```python
from build123d import *

# Parameters (mm, degrees)
SKETCH2_R               = 2.15
BOSS_EXTRUDE1_DEPTH     = 12.7
CUT_EXTRUDE1_DEPTH      = 86.777857097
CUT_EXTRUDE1_DEPTH_BACK = 86.777857097
SKETCH3_W               = 5.08
SKETCH3_H               = 2.54
BOSS_EXTRUDE2_DEPTH     = 12.7
SKETCH5_R               = 9.75
CUT_EXTRUDE2_DEPTH      = 5.5
CUT_EXTRUDE3_DEPTH      = 90.593664183
CUT_EXTRUDE3_DEPTH_BACK = 90.593664183
SKETCH6_R               = 1.25


with BuildPart() as part:
    # Sketch2 → Boss-Extrude1 (new body)
    with BuildSketch(Plane(origin=(0, 0, 0), x_dir=(1, 0, 0), z_dir=(0, 1, 0))):
        with BuildLine():
            Line((0, 8.382), (74.7776, 8.382))
            ThreePointArc((74.7776, 8.382), (83.1596, 0), (74.7776, -8.382))
            Line((74.7776, -8.382), (0, -8.382))
            ThreePointArc((0, -8.382), (-8.382, 0), (0, 8.382))
        make_face()
        with Locations(Location((0, 0, 0), (0, 0, 270))):
            Circle(SKETCH2_R, mode=Mode.SUBTRACT)
        with Locations(Location((74.7776, 0, 0), (0, 0, 270))):
            Circle(SKETCH2_R, mode=Mode.SUBTRACT)
    extrude(amount=-BOSS_EXTRUDE1_DEPTH)

    # Sketch3 → Cut-Extrude1 (cut, two sides: drawn at the far end of the back side and taken through both)
    with BuildSketch(Plane(origin=(0, 0, -8.382), x_dir=(-1, 0, 0), z_dir=(0, 0, -1)).offset(-CUT_EXTRUDE1_DEPTH_BACK)):
        with Locations((-43.750123937, -4.528631303)):
            Rectangle(SKETCH3_W, SKETCH3_H)
    extrude(amount=CUT_EXTRUDE1_DEPTH + CUT_EXTRUDE1_DEPTH_BACK, mode=Mode.SUBTRACT)

    # Sketch4 → Boss-Extrude2 (add)
    with BuildSketch(Plane(origin=(0, 0, 0), x_dir=(1, 0, 0), z_dir=(0, 1, 0))):
        with BuildLine():
            Line((71.377269841, 13.064752382), (70.480233935, 12.79775937))
            ThreePointArc((70.480233935, 12.79775937), (67.016909963, 11.04634284), (64.194969136, 8.382))
            Line((64.194969136, 8.382), (74.7776, 8.382))
            ThreePointArc((74.7776, 8.382), (83.1596, 0), (74.7776, -8.382))
            Line((74.7776, -8.382), (64.194969136, -8.382))
            ThreePointArc((64.194969136, -8.382), (66.930768284, -10.985318931), (70.280616628, -12.728988198))
            ThreePointArc((70.280616628, -12.728988198), (82.573134763, -11.021780154), (88.2776, 0))
            ThreePointArc((88.2776, 0), (83.034280412, 10.680694199), (71.377269841, 13.064752382))
        make_face()
        with BuildLine():
            Line((70.480233935, 12.79775937), (55.644284932, 8.382))
            Line((55.644284932, 8.382), (64.194969136, 8.382))
            ThreePointArc((64.194969136, 8.382), (67.016909963, 11.04634284), (70.480233935, 12.79775937))
        make_face()
        with BuildLine():
            ThreePointArc((70.280616628, -12.728988198), (66.930768284, -10.985318931), (64.194969136, -8.382))
            Line((64.194969136, -8.382), (55.644284932, -8.382))
            Line((55.644284932, -8.382), (70.280616628, -12.728988198))
        make_face()
    extrude(amount=-BOSS_EXTRUDE2_DEPTH)

    # Sketch5 → Cut-Extrude2 (cut)
    with BuildSketch(Plane(origin=(0, -12.7, 0), x_dir=(-1, 0, 0), z_dir=(0, -1, 0))):
        with Locations(Location((-74.7776, 0, 0), (0, 0, 90))):
            Circle(SKETCH5_R)
    extrude(amount=-CUT_EXTRUDE2_DEPTH, mode=Mode.SUBTRACT)

    # Sketch6 → Cut-Extrude3 (cut, two sides: drawn at the far end of the back side and taken through both)
    with BuildSketch(Plane(origin=(0, -7.2, 0), x_dir=(-1, 0, 0), z_dir=(0, -1, 0)).offset(-CUT_EXTRUDE3_DEPTH_BACK)):
        with Locations(Location((-74.876863781, 6.35, 0), (0, 0, 90))):
            Circle(SKETCH6_R)
        with Locations(Location((-68.4276, 0.099263781, 0), (0, 0, 90))):
            Circle(SKETCH6_R)
        with Locations(Location((-74.678336219, -6.35, 0), (0, 0, 90))):
            Circle(SKETCH6_R)
        with Locations(Location((-81.1276, -0.099263781, 0), (0, 0, 90))):
            Circle(SKETCH6_R)
    extrude(amount=CUT_EXTRUDE3_DEPTH + CUT_EXTRUDE3_DEPTH_BACK, mode=Mode.SUBTRACT)


solid = part.part
```
Geometry: final body of the model. Coordinates: model frame, mm. A direction names the side the tool comes from. Give positions to 0.01 mm unless a question says otherwise; leave off trailing zeros. Write each loop counter-clockwise with the first axis right and the second up, starting at its lowest first coordinate (ties: lowest second). Pieces come first, ordered by that corner, then holes.
1. Reachability of faces 4 (the flat face through (27, -6, -8.382)), 5 (the flat face through (46.29, -5, 0)), 6 (the flat face through (39, -12.7, 0)), 7 (the flat face through (74.9, -7.2, 2.3)), 8 (the flat face through (28, -6, 8.382)) from +Z, -Z, +X, -X, +Y, -Y: full face, straight path, thin tool, end or side. Return the list, or none.
2. Pin query (flat end, axial travel): P1, Ø4, axis at x = 42, y = -8.5, coming from the -Z side; P2, Ø2, axis at x = 68.43, z = -0.1, coming from the -Y side; P3, Ø4, axis at x = 40, y = -3.5, coming from the +Z side; P4, Ø2, axis at y = -8, z = -6.5, coming from the +X side. Return the tip coordinate at first contact, or that it passes through.
3. Line query: probe 1 along X at (y, z) = (-9.5, 0); probe 2 along Z at (x, y) = (33.5, -11.75); probe 3 along X at (y, z) = (-3.75, 6.35). Output: solid intervals per line, ascending.
4. Draft query along X for faces 1 (the flat face through (39, 0, 0)), 2 (the cylindrical face through (83, -9.99, -5.24)), 3 (the cylindrical face through (-8.38, -6.26, 0.18)). Return one class per face: released by +X, released by -X, zero draft, split by the parting line, or undercut.
5. Section query B-B, the plane y = -4.25. Return loops of the section in (x, z).
6. Section query A-A, the plane z = 6.35. Return loops of the section in (x, y).
7. Section query C-C, the plane y = -8.75. Return loops of the section in (x, z).
8. Section query D-D, the plane x = 51.5. Return loops of the section in (y, z).
Computed:
1. face 4: -Z, -X, +Y, -Y
1. face 5: +Z, -Z
1. face 6: +Z, -Z, +X, -X, -Y
1. face 7: -Y
1. face 8: +Z, -X, +Y, -Y
2. P1: stops at z = -8.38
2. P2: passes through
2. P3: stops at z = 8.38
2. P4: stops at x = 87.11
3. probe 1: x = -8.38 to -2.15, 2.15 to 65.03, 84.53 to 88.28
3. probe 2: z = -8.38 to 8.38
3. probe 3: x = -5.47 to 41.21, 46.29 to 73.43, 75.93 to 86.69
4. face 1: zero draft
4. face 2: undercut
4. face 3: released by -X
5. outline: (0, -8.38) - (41.21, -8.38) - (41.21, 8.38) - (0, 8.38) arc R8.38 ccw to start; (46.29, -8.38) - (55.64, -8.38) - (71.38, -13.06) arc R13.5 ccw (long way) to (70.28, 12.73) - (55.64, 8.38) - (46.29, 8.38) - close; hole circle Ø4.3 at (0, 0); hole circle Ø2.5 at (68.43, -0.1); hole circle Ø4.3 at (74.78, 0); hole circle Ø2.5 at (74.68, 6.35); hole circle Ø2.5 at (74.88, -6.35); hole circle Ø2.5 at (81.13, 0.1)
6. outline: (-5.47, -12.7) - (67.38, -12.7) - (67.38, -7.2) - (73.43, -7.2) - (73.43, 0) - (-5.47, 0) - close; (75.93, -7.2) - (82.18, -7.2) - (82.18, -12.7) - (86.69, -12.7) - (86.69, 0) - (75.93, 0) - close; hole (41.21, -5.8) - (46.29, -5.8) - (46.29, -3.26) - (41.21, -3.26) - close
7. outline: (0, -8.38) - (55.64, -8.38) - (71.38, -13.06) arc R13.5 ccw (long way) to (70.28, 12.73) - (55.64, 8.38) - (0, 8.38) arc R8.38 ccw to start; hole circle Ø4.3 at (0, 0); hole circle Ø19.5 at (74.78, 0)
8. outline: (-12.7, -8.38) - (0, -8.38) - (0, 8.38) - (-12.7, 8.38) - close
